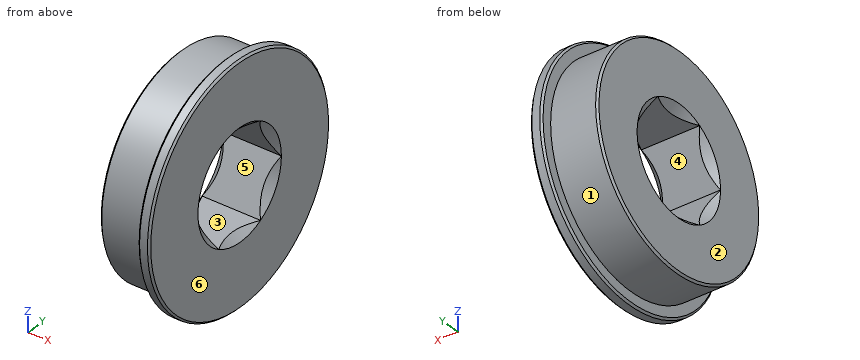
from build123d import *

# Parameters (mm, degrees)
CUT_EXTRUDE1_DEPTH = 8.9248
CHAMFER1_SIZE      = 0.254


with BuildPart() as part:
    # Sketch1 → Revolve1 (revolve)
    with BuildSketch(Plane.XY):
        Polygon((-3.9624, 14.2875), (2.3876, 14.2875), (2.3876, 15.875), (3.9624, 15.875), (3.9624, 7.332348419), (2.980051581, 6.35), (-2.980051581, 6.35), (-3.9624, 7.332348419), align=None)
    revolve(axis=Axis((3.9624, 0, 0), (-1, 0, 0)))

    # Sketch2 → Cut-Extrude1 (cut, through all)
    with BuildSketch(Plane(origin=(3.9624, 0, 0), x_dir=(0, 0, -1), z_dir=(1, 0, 0))):
        Polygon((0, 7.332348419), (-6.35, 3.666174209), (-6.35, -3.666174209), (0, -7.332348419), (6.35, -3.666174209), (6.35, 3.666174209), align=None)
    extrude(amount=-CUT_EXTRUDE1_DEPTH, mode=Mode.SUBTRACT)

    # Chamfer1
    chamfer1_edges = [part.edges().sort_by_distance(p)[0] for p in [
        (3.9624, -15.875, 0),
        (2.3876, -15.875, 0),
        (-3.9624, -14.2875, 0),
    ]]
    chamfer(chamfer1_edges, length=CHAMFER1_SIZE)


solid = part.part
Could you check a few things on this model? Use its own coordinates, in mm. Face numbers are marked on the shaded views. A direction names the side the tool comes from. Round coordinates to 2 decimals unless told otherwise and drop trailing zeros. Put each result on its own line as item: value. Start each with the question number.
(1) For the marked faces 5 and 6, which set-ups out of +Z, -Z, +X, -X, +Y, -Y let a thin tool reach every point of the face, with its end or its side?
(2) Thinking about a two-plate mould opening in Y: for the marked faces 1, 2, 3 and 4, which applies, released by +Y, released by -Y, zero draft, split by the parting line, or undercut?
(3) Will these pins go through, and if not, where does the flat tip stop? pin 1 (3 mm diameter, centred on x = 0.5, z = 9.5, fed in from +Y); pin 2 (2 mm diameter, centred on x = -0.5, y = 10, fed in from +Z); pin 3 (2 mm diameter, centred on y = 2.5, z = -4.5, fed in from -X); pin 4 (4 mm diameter, centred on y = 3, z = 4, fed in from -X).
(4) I need wall thicknesses on probe 1 along Z at (x, y) = (2.5, -2.5); probe 2 along Z at (x, y) = (1, -6.5); probe 3 along Y at (x, z) = (-1, 1) (3 decimals). Which ranges of each line are inside material? Lowest first, please.
Here are the results:
1. face 5: +X, -X
1. face 6: +Z, -Z, +X, +Y, -Y
2. face 1: split by the parting line
2. face 2: zero draft
2. face 3: undercut
2. face 4: undercut
3. pin 1: stops at y = 11.84
3. pin 2: stops at z = 11.1
3. pin 3: passes through
3. pin 4: stops at x = -3.63
4. probe 1: z = -15.53 to -6.35, 6.35 to 15.53
4. probe 2: z = -12.72 to -1.44, 1.44 to 12.72
4. probe 3: y = -14.252 to -6.755, 6.755 to 14.252
